The listing builds one solid part. Answer for the finished solid, in the listing's coordinates (mm). A direction names the side the tool comes from. Coordinates: 2 decimals unless noted, no trailing zeros. Order: outer loops, then holes, each group sorted by start corner. A loop starts at its lowest first (then second) coordinate and runs counter-clockwise, first axis right, second up. Notation, with made-up numbers: (-33.5, 86) -> (19.5, 86) arc R7 ccw to (19.5, 92) -> close; hole circle Ø6 at (34, 70). An arc over 180 degrees is marked (long way). Return JSON: item names as keys, results as strings.
```python
from build123d import *

# Parameters (mm, degrees)
SKETCH1_R           = 1.905
SKETCH1_W           = 12.7
SKETCH1_H           = 3.175
BOSS_EXTRUDE1_DEPTH = 3.175


with BuildPart() as part:
    # Sketch1 → Boss-Extrude1 (new body)
    with BuildSketch(Plane(origin=(0, 0, 0), x_dir=(1, 0, 0), z_dir=(0, 1, 0))):
        Polygon((-38.1, 6.604), (-34.925, 6.604), (-34.925, 8.8265), (-32.385, 8.8265), (-32.385, 6.604), (-27.305, 6.604), (-27.305, 3.175), (-32.385, 3.175), (-32.385, 0.9525), (-34.925, 0.9525), (-34.925, 3.175), (-38.1, 3.175), (-38.1, 0), (0, 0), (38.1, 0), (38.1, 3.175), (34.925, 3.175), (34.925, 0.9525), (32.385, 0.9525), (32.385, 3.175), (27.305, 3.175), (27.305, 6.604), (32.385, 6.604), (32.385, 8.8265), (34.925, 8.8265), (34.925, 6.604), (38.1, 6.604), (38.1, 155.5115), (34.925, 155.5115), (34.925, 153.3525), (32.385, 153.3525), (32.385, 155.5115), (27.94, 155.5115), (27.94, 159.0675), (32.385, 159.0675), (32.385, 161.2265), (34.925, 161.2265), (34.925, 159.0675), (38.1, 159.0675), (38.1, 166.8145), (-38.1, 166.8145), (-38.1, 159.0675), (-34.925, 159.0675), (-34.925, 161.2265), (-32.385, 161.2265), (-32.385, 159.0675), (-27.94, 159.0675), (-27.94, 155.5115), (-32.385, 155.5115), (-32.385, 153.3525), (-34.925, 153.3525), (-34.925, 155.5115), (-38.1, 155.5115), align=None)
        with Locations(Location((-34.925, 42.9895, 0), (0, 0, 270))):
            Circle(SKETCH1_R, mode=Mode.SUBTRACT)
        with Locations(Location((-34.925, 147.7645, 0), (0, 0, 270))):
            Circle(SKETCH1_R, mode=Mode.SUBTRACT)
        with Locations(Location((34.925, 42.9895, 0), (0, 0, 270))):
            Circle(SKETCH1_R, mode=Mode.SUBTRACT)
        with Locations(Location((34.925, 147.7645, 0), (0, 0, 270))):
            Circle(SKETCH1_R, mode=Mode.SUBTRACT)
        with Locations((-15.875, 31.877)):
            Rectangle(SKETCH1_W, SKETCH1_H, mode=Mode.SUBTRACT)
        with Locations((15.875, 31.877)):
            Rectangle(SKETCH1_W, SKETCH1_H, mode=Mode.SUBTRACT)
        with BuildLine():
            Line((9.525, 150.9395), (9.525, 122.3645))
            ThreePointArc((9.525, 122.3645), (0, 112.8395), (-9.525, 122.3645))
            Line((-9.525, 122.3645), (-9.525, 150.9395))
            ThreePointArc((-9.525, 150.9395), (0, 160.4645), (9.525, 150.9395))
        make_face(mode=Mode.SUBTRACT)
    extrude(amount=BOSS_EXTRUDE1_DEPTH)


solid = part.part
```
Item 1: Determine the mould class of faces 1 (the flat face through (-38.1, 2, -163)), 2 (the flat face through (36, 2, -159.068)), 3 (the flat face through (9.525, 2, -32)) for opening direction Z: pulls with the +Z half, pulls with the -Z half, needs draft (parallel to the pull), parting line crosses it, or undercut.
Answer list:
{"face 1": "needs draft", "face 2": "undercut", "face 3": "undercut"}
Item 2: Flat-ended cylindrical pins translate along their axes: pin 1 (1.6 mm diameter, centred on y = 1.5, z = -5.5, fed in from +X) (3 decimals); pin 2 (3 mm diameter, centred on x = -34.92, z = -147.76, fed in from +Y). Find the tip coordinate at first contact, or state that the pin passes through.
Answer list:
{"pin 1": "x = 27.305", "pin 2": "through"}
Item 3: The part is cut by section A-A on x = -18. Determine the outline of the cut face in (y, z) (1 decimal), plus the area to 3 significant figures.
Answer list:
{"outline": "(0, -166.8) -> (3.2, -166.8) -> (3.2, -33.5) -> (0, -33.5) -> close; (0, -30.3) -> (3.2, -30.3) -> (3.2, 0) -> (0, 0) -> close", "area": "520 mm2"}
Item 4: The part is cut by section C-C on y = 1.65. Count the separate pieces of the cut face and the enclosed holes in it, plus the area to 3 significant figures.
Answer list:
{"separate pieces": "1", "enclosed holes": "7", "area": "11,600 mm2"}
Item 5: Find the intervals of material crossed by probe 1 along Z at (x, y) = (-30, 3) (1 decimal); probe 2 along X at (y, z) = (1.1, -137) (3 decimals); probe 3 along Z at (x, y) = (-27.5, 0.45) (1 decimal), in increasing order.
Answer list:
{"probe 1": "-166.8 to -159.1, -155.5 to -6.6, -3.2 to 0", "probe 2": "-38.1 to -9.525, 9.525 to 38.1", "probe 3": "-166.8 to -6.6, -3.2 to 0"}
Item 6: The part is cut by section B-B on x = 0. Determine the outline of the cut face in (y, z) (1 decimal), plus the area to 3 significant figures.
Answer list:
{"outline": "(0, -166.8) -> (3.2, -166.8) -> (3.2, -160.5) -> (0, -160.5) -> close; (0, -112.8) -> (3.2, -112.8) -> (3.2, 0) -> (0, 0) -> close", "area": "378 mm2"}
Item 7: Which of the six approach directions +Z, -Z, +X, -X, +Y, -Y give full straight-line access (tool end or side, diameter ignored) to faces 4 (the flat face through (22.225, 2, -32)), 5 (the flat face through (-30, 2, -159.068)), 6 (the flat face through (27.94, 2, -157))?
Answer list:
{"face 4": "+Y, -Y", "face 5": "-X, +Y, -Y", "face 6": "+X, +Y, -Y"}
